Read the model definition and answer for the solid it produces. Units are mm, in the model's axes. A direction names the side the tool comes from. Round coordinates to 2 decimals unless told otherwise and drop trailing zeros. Order: outer loops, then holes, each group sorted by start corner. A loop starts at its lowest first (then second) coordinate and runs counter-clockwise, first axis right, second up. Notation, with made-up numbers: (-24.5, 47) - (-18.5, 47) arc R25 ccw to (-18.5, 66) - close; hole circle Ø5 at (-17.5, 18). An arc over 180 degrees is marked (long way). Answer as a JSON object with one key per item and string values. Group by question number.
Q1. A cutting plane is placed at D-D on x = -18. Determine the outline of the cut face in (y, z) (3 decimals).
Q2. A cutting plane is placed at C-C on z = -22. Determine the outline of the cut face in (x, y) (3 decimals), and give its area (3 significant figures).
Q3. Given pin 1 Ø10 at (y, z) = (5.5, -15.5) entering from +X; pin 2 Ø3 at (x, z) = (-7.5, -19) entering from +Y (3 decimals); pin 3 Ø6.5 at (x, y) = (-23.5, 16) entering from -Z (3 decimals), each flat-ended and moving along its own axis, determine where each tip first touches the part or whether it passes through.
Q4. Consider line 1 (Y direction, x = -25.4, z = -1.7) (3 decimals); line 2 (Y direction, x = -33, z = -19.75) (3 decimals); line 3 (Z direction, x = -37, y = 23.25) (3 decimals). Determine where each line is inside the solid, lowest interval first.
Q5. The mould has two halves that part along Y. Classify faces 3 (the cylindrical face through (-26.865, 16.233, -1.61)), 4 (the flat face through (-26, 25.4, -2)), 5 (the flat face through (-26, 2, -25.4)), 6 (the flat face through (-25, 0, -13)): pulls with the +Y half, pulls with the -Y half, needs draft (parallel to the pull), parting line crosses it, or undercut.
Q6. A cutting plane is placed at B-B on y = 19.05. Determine the outline of the cut face in (x, z) (3 decimals), and give its area (3 significant figures).
Q7. A tool of negligible diameter and unlimited length cuts with its end or side. For faces 1 (the flat face through (-25, 3.175, -14)), 2 (the flat face through (0, 2, -8)), from which of +Z, -Z, +X, -X, +Y, -Y can it reach the whole face along a straight path? Write none if from no direction.
Q8. A cutting plane is placed at A-A on x = -25.4. Determine the outline of the cut face in (y, z) (3 decimals).
Autodesk Inventor part; units mm, degrees
ref_plane "YZ Plane" through (0, 0, 0) normal (1, 0, 0) x (0, 1, 0)
ref_plane "XZ Plane" through (0, 0, 0) normal (0, 1, 0) x (-1, 0, 0)
ref_plane "XY Plane" through (0, 0, 0) normal (0, 0, 1) x (1, 0, 0)
sketch "Sketch1" plane through (0, 0, 0) normal (0, 1, 0) x (-1, 0, 0)
  line L0 (0, 0) -> (50.8, 0)
  line L1 (50.8, 0) -> (50.8, -25.4)
  line L2 (50.8, -25.4) -> (0, -25.4)
  line L3 (0, -25.4) -> (0, 0)
  dimension "d0" = 50.8
  dimension "d1" = 25.4
extrude "Extrusion1" add sketch "Sketch1" along normal blind 3.175
sketch "Sketch2" plane through (0, 3.175, 0) normal (0, 1, 0) x (1, 0, 0)
  line L0 (-50.8, 0) -> (0, 0)
  line L1 (0, 0) -> (0, 3.175)
  line L2 (0, 3.175) -> (-50.8, 3.175)
  line L3 (-50.8, 3.175) -> (-50.8, 0)
  dimension "d4" = 50.8
  dimension "d5" = 3.175
extrude "Extrusion2" add sketch "Sketch2" along normal blind 22.225
sketch "Sketch3" plane through (0, 3.175, -3.175) normal (0, 0, -1) x (-1, 0, 0)
  circle A0 centre (25.4, 15.875) radius 3.175
  line L0 (0, 22.225) -> (50.8, 22.225)
  line L1 (50.8, 0) -> (50.8, 22.225)
  point P0 (0, -3.175)
  dimension "d8" = 6.35
  dimension "d9" = 6.35
  dimension "d10" = 25.4
extrude "Extrusion3" cut sketch "Sketch3" against normal through all
properties part number "Gusset"
Result set:
{
 "1": {"outline": "(0, -25.4) - (3.175, -25.4) - (3.175, -3.175) - (25.4, -3.175) - (25.4, 0) - (0, 0) - close"},
 "2": {"outline": "(-50.8, 0) - (0, 0) - (0, 3.175) - (-50.8, 3.175) - close", "area": "161 mm²"},
 "3": {"pin 1": "stops at x = 0", "pin 2": "stops at y = 3.175", "pin 3": "stops at z = -3.175"},
 "4": {"line 1": "y = 0 to 15.875, 22.225 to 25.4", "line 2": "y = 0 to 3.175", "line 3": "z = -3.175 to 0"},
 "5": {"face 3": "undercut", "face 4": "pulls with the +Y half", "face 5": "needs draft", "face 6": "pulls with the -Y half"},
 "6": {"outline": "(-50.8, -3.175) - (-28.575, -3.175) - (-28.575, 0) - (-50.8, 0) - close; (-22.225, -3.175) - (0, -3.175) - (0, 0) - (-22.225, 0) - close", "area": "141 mm²"},
 "7": {"face 1": "-Z, +X, -X, +Y", "face 2": "+Z, -Z, +X, +Y, -Y"},
 "8": {"outline": "(0, -25.4) - (3.175, -25.4) - (3.175, -3.175) - (15.875, -3.175) - (15.875, 0) - (0, 0) - close; (22.225, -3.175) - (25.4, -3.175) - (25.4, 0) - (22.225, 0) - close"}
}
